Here's the drawing with two shaded views (mm, measured from the low corner). I have some questions. Round coordinates to 2 decimals unless told otherwise and drop trailing zeros. Loops run counter-clockwise (first coordinate to the right, second up) from the corner with the lowest first, then second, coordinate; pieces in that order, holes last. Notation, with made-up numbers: M -10,83.5 L 6,83.5 A29 ccw 6,121.5 Z; hole C 27.5,-38.75 d8. An arc over 180 degrees is marked long. Answer as a JSON object with one key per item and string values.
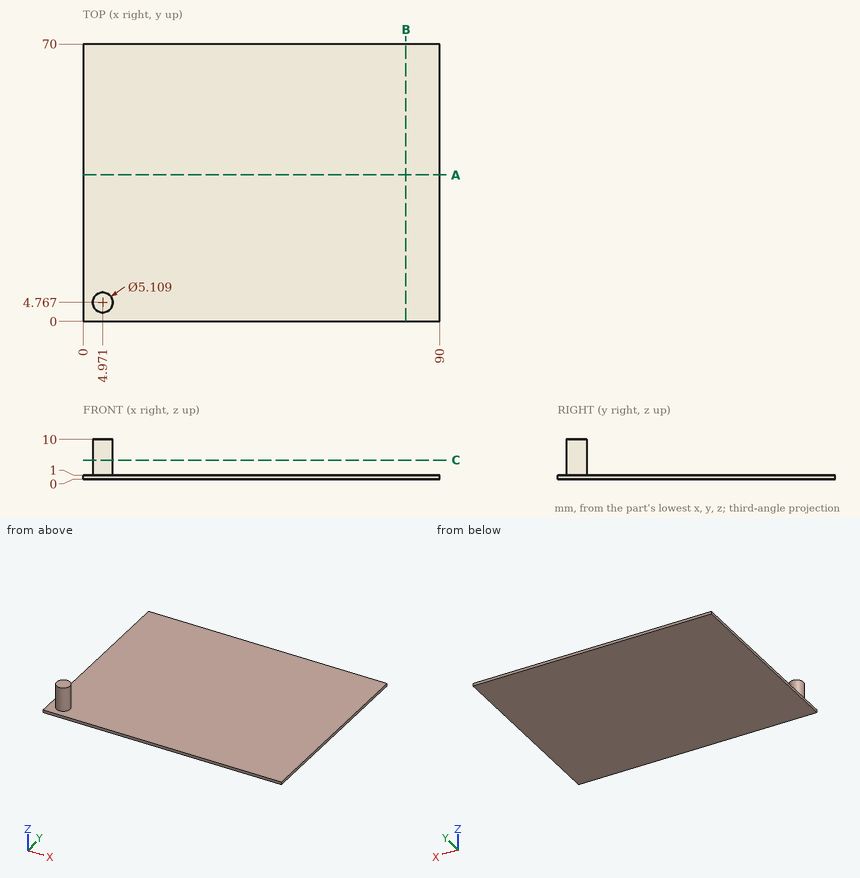
Item 1: I want a section at B-B on x = 81.5. List the corners of the cut face in (y, z) for me.
Solution:
{"outline": "M 0,0 L 70,0 L 70,1 L 0,1 Z"}
Item 2: If I drill on L1, parallel to Z at x = 18, y = 14; L2, parallel to X at y = 5, z = 8.75 (1 decimal), over which ranges is the centre line in solid material (lowest first)? Write a range as from..to.
Solution:
{"L1": "z = 0..1", "L2": "x = 2.4..7.5"}
Item 3: For P1, Ø4, axis at x = 42.5, y = 20.5, coming from the +Z side, with a flat end and sliding along its axis, tell me the tip position at first contact or that it passes through.
Solution:
{"P1": "stops at z = 1"}
Item 4: I want a section at A-A on y = 37. List the corners of the cut face in (x, z) for me.
Solution:
{"outline": "M 0,0 L 90,0 L 90,1 L 0,1 Z"}
Item 5: I want a section at C-C on z = 4.75. List the corners of the cut face in (x, y) for me (1 decimal), plus the area to 3 significant figures.
Solution:
{"outline": "C 5,4.8 d5.1", "area": "20.5 mm2"}
